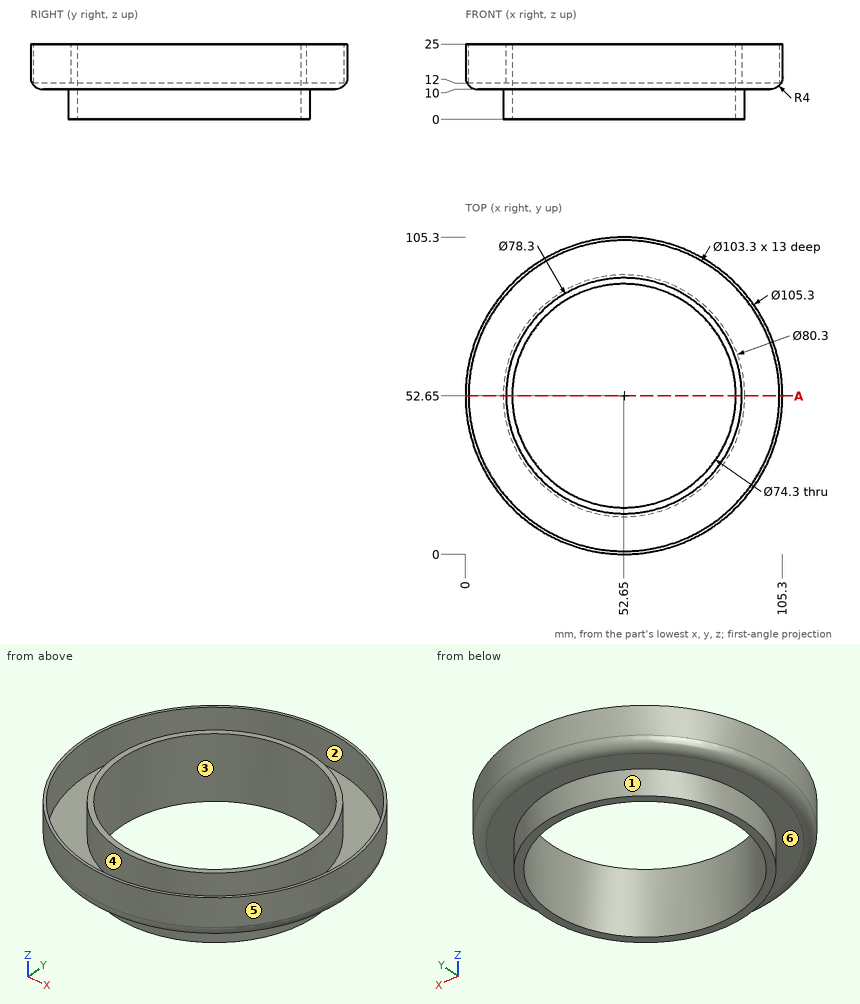
Verification items for this drawing (mm, ordinates from the low corner). A direction names the side the tool comes from. Coordinates: 2 decimals unless noted, no trailing zeros. Write each loop counter-clockwise with the first axis right and the second up, starting at its lowest first coordinate (ties: lowest second). Pieces come first, ordered by that corner, then holes. Notation, with made-up numbers: M 79,-35 L 99,-35 A21 cw 99,-3 Z; hole C 54.25,79 d2. An arc over 180 degrees is marked long. Use one line per item in the form item = value. Start each with the question number.
1) Set-up check for the marked faces 1, 2 and 3: record each of +Z, -Z, +X, -X, +Y, -Y from which the full face is reachable in a straight line by a thin tool's end or side.
2) Go/stop test with flat-tipped pins: pin 1 Ø8 at (y, z) = (44, 22) entering from +X; pin 2 Ø10 at (x, z) = (43.5, 14.5) entering from +Y; pin 3 Ø8 at (x, z) = (45, 16.5) entering from -Y. Record where each tip stops, or that it passes through.
3) Section check A-A on y = 52.65. Enter the section's corners in (x, z), and give its area (3 significant figures).
4) Thickness scan on probe 1 along Y at (x, z) = (52.65, 17.5); probe 2 along X at (y, z) = (44, 12.25); probe 3 along Y at (x, z) = (77, 23.25). Record the ranges inside material, lowest first. Write a range as from..to.
5) Release check for a two-part mould opening along Y. For the marked faces 4, 5 and 6 record: pulls with the +Y half, pulls with the -Y half, needs draft (parallel to the pull), parting line crosses it, or undercut.
Responses:
q1.face_1 = -Z
q1.face_2 = +Z
q1.face_3 = +Z, -Z
q2.pin_1 = 105.09
q2.pin_2 = 105.14
q2.pin_3 = 0.13
q3.outline = M 0,14 A4 ccw 4,10 L 12.5,10 L 12.5,0 L 15.5,0 L 15.5,25 L 13.5,25 L 13.5,12 L 1,12 L 1,25 L 0,25 Z; M 89.8,0 L 92.8,0 L 92.8,10 L 101.3,10 A4 ccw 105.3,14 L 105.3,25 L 104.3,25 L 104.3,12 L 91.8,12 L 91.8,25 L 89.8,25 Z
q3.area = 193 mm2
q4.probe_1 = 0..1, 13.5..15.5, 89.8..91.8, 104.3..105.3
q4.probe_2 = 1.12..1.73, 14.47..16.52, 88.78..90.83, 103.57..104.18
q4.probe_3 = 5.97..7.1, 21.99..24.59, 80.71..83.31, 98.2..99.33
q5.face_4 = undercut
q5.face_5 = parting line crosses it
q5.face_6 = needs draft
